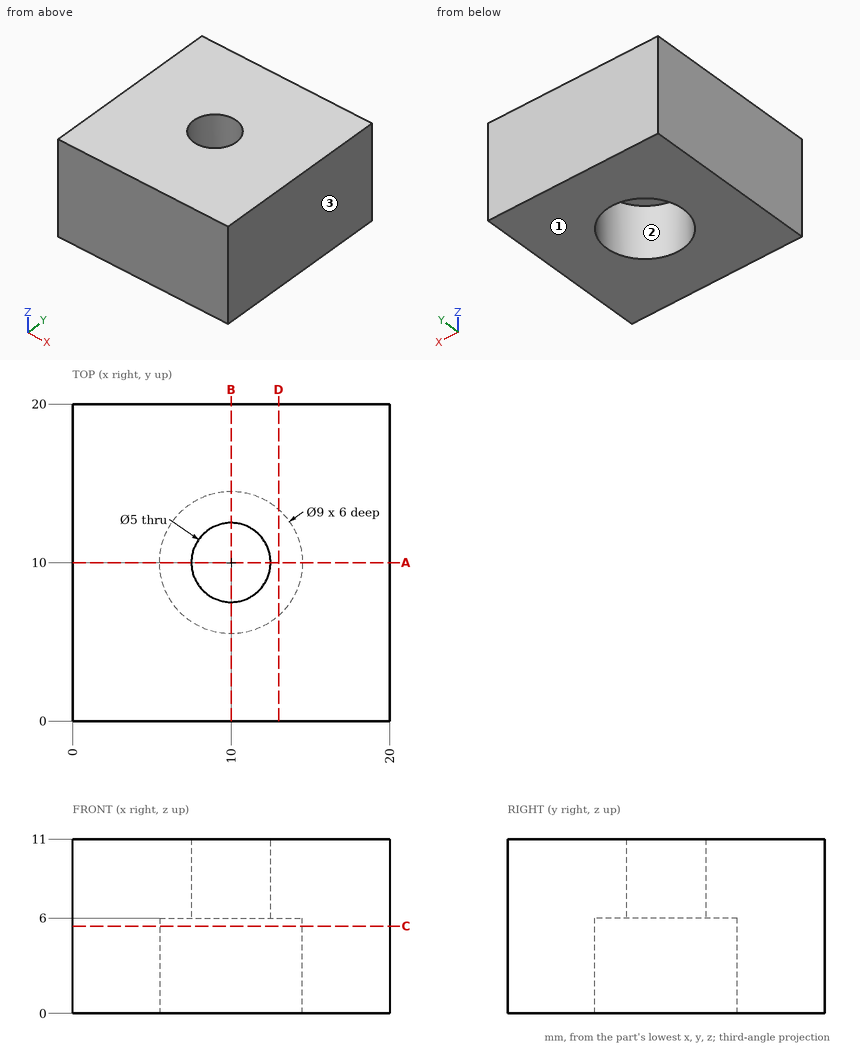
Here's the drawing with two shaded views (mm, measured from the low corner). I have some questions. Coordinates: 2 decimals unless noted, no trailing zeros. Order: outer loops, then holes, each group sorted by start corner. A loop starts at its lowest first (then second) coordinate and runs counter-clockwise, first axis right, second up.
Item 1: If we mould it in two halves opening along X, with no side actions, what happens to the marked faces 1, 2 and 3? For each: +X half, -X half, draft (parallel to the pull), parting line (faces both ways), or undercut.
Result sheet:
face 1: draft
face 2: undercut
face 3: +X half
Item 2: If we section it at A-A on y = 10: List the corners of the cut face in (x, z) for me.
Result sheet:
outline: (0, 0) - (5.5, 0) - (5.5, 6) - (7.5, 6) - (7.5, 11) - (0, 11) - close; (12.5, 6) - (14.5, 6) - (14.5, 0) - (20, 0) - (20, 11) - (12.5, 11) - close
Item 3: I need wall thicknesses on line 1 (Y direction, x = 10, z = 8.2); line 2 (Z direction, x = 11.5, y = 12.5); line 3 (Y direction, x = 7.25, z = 1.5). Which ranges of each line are inside material? Lowest first, please.
Result sheet:
line 1: y = 0 to 7.5, 12.5 to 20
line 2: z = 6 to 11
line 3: y = 0 to 6.44, 13.56 to 20
Item 4: If we section it at D-D on x = 13: List the corners of the cut face in (y, z) for me, plus the area to 3 significant figures.
Result sheet:
outline: (0, 0) - (6.65, 0) - (6.65, 6) - (13.35, 6) - (13.35, 0) - (20, 0) - (20, 11) - (0, 11) - close
area: 180 mm2
Item 5: If we section it at C-C on z = 5.5: List the corners of the cut face in (x, y) for me, plus the area to 3 significant figures.
Result sheet:
outline: (0, 0) - (20, 0) - (20, 20) - (0, 20) - close; hole circle Ø9 at (10, 10)
area: 336 mm2
